from build123d import *

# Parameters (mm, degrees)
BOSS_EXTRUDE1_DEPTH     = 40
SKETCH2_R               = 1.5
CUT_EXTRUDE1_DEPTH      = 1
CUT_EXTRUDE1_DEPTH_BACK = 12
CHAMFER1_SIZE           = 0.2
SKETCH4_R               = 1.5
BOSS_EXTRUDE2_DEPTH     = 6.5
CHAMFER2_SIZE           = 0.6


with BuildPart() as part:
    # Sketch1 → Boss-Extrude1 (new body)
    with BuildSketch(Plane.XY):
        Polygon((2.621170222, 0), (1.310585111, 2.27), (-1.310585111, 2.27), (-2.621170222, 0), (-1.310585111, -2.27), (1.310585111, -2.27), align=None)
    extrude(amount=BOSS_EXTRUDE1_DEPTH)

    # Sketch2 → Cut-Extrude1 (cut, two sides)
    with BuildSketch(Plane.XY.offset(40)) as cut_extrude1_sk:
        Circle(SKETCH2_R)
    extrude(amount=CUT_EXTRUDE1_DEPTH, mode=Mode.SUBTRACT)
    extrude(cut_extrude1_sk.sketch, amount=-CUT_EXTRUDE1_DEPTH_BACK, mode=Mode.SUBTRACT)

    # Sketch3 → Cut-Revolve1 (revolve, cut)
    with BuildSketch(Plane(origin=(0, 0, 0), x_dir=(1, 0, 0), z_dir=(0, 1, 0))):
        Polygon((-2.621170222, -40), (-2.271170222, -40), (-2.621170222, -39.8), align=None)
    revolve(axis=Axis((0, 0, 28), (0, 0, 1)), mode=Mode.SUBTRACT)

    # Chamfer1
    chamfer1_edges = [part.edges().sort_by_distance(p)[0] for p in [
        (-1.5, 0, 40),
    ]]
    chamfer(chamfer1_edges, length=CHAMFER1_SIZE)

    # Sketch4 → Boss-Extrude2 (add)
    with BuildSketch(Plane(origin=(0, 0, 0), x_dir=(-1, 0, 0), z_dir=(0, 0, -1))):
        Circle(SKETCH4_R)
    extrude(amount=BOSS_EXTRUDE2_DEPTH)

    # Chamfer2
    chamfer2_edges = [part.edges().sort_by_distance(p)[0] for p in [
        (1.5, 0, -6.5),
    ]]
    chamfer(chamfer2_edges, length=CHAMFER2_SIZE)


solid = part.part
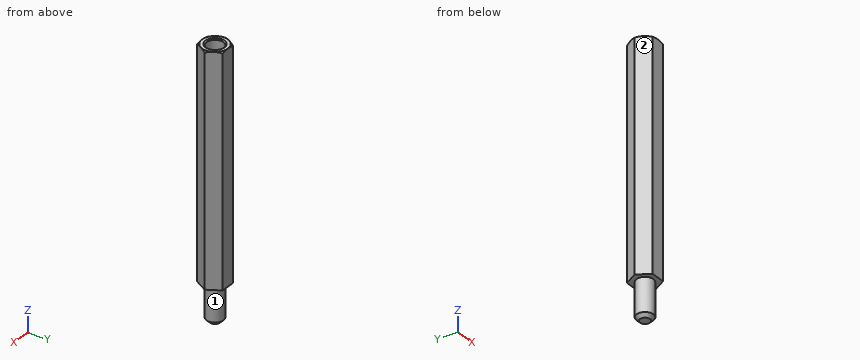
Geometry check sheet. Reference: the model listing, model coordinates, mm. Face numbers are marked on the shaded views. A direction names the side the tool comes from. Coordinates: 2 decimals unless noted, no trailing zeros. Write each loop counter-clockwise with the first axis right and the second up, starting at its lowest first coordinate (ties: lowest second). Pieces come first, ordered by that corner, then holes. Notation, with made-up numbers: (-0.5, -16) -> (27.5, -16) arc R23 cw to (27.5, 17) -> close; hole circle Ø3 at (28.5, 0). An arc over 180 degrees is marked (long way). One line per question, with ' | ' between items.
1. Depth check by flat-ended pin: pin 1 Ø1.5 at (x, y) = (2, -1.5) entering from +Z; pin 2 Ø0.9 at (x, y) = (-0.5, 0) entering from +Z. Enter the tip coordinate at first touch or a pass-through.
Answers:
pin 1: stops at z = 40 | pin 2: stops at z = 28
2. Cross-section at A-A on z = 6. Record the cut outline in (x, y), and give its area (3 significant figures).
Answers:
outline: (-2.62, 0) -> (-1.31, -2.27) -> (1.31, -2.27) -> (2.62, 0) -> (1.31, 2.27) -> (-1.31, 2.27) -> close | area: 17.9 mm²
3. Set-up check for the marked faces 1 and 2: record each of +Z, -Z, +X, -X, +Y, -Y from which the full face is reachable in a straight line by a thin tool's end or side.
Answers:
face 1: -Z | face 2: +Z, -Z, -X, -Y
4. Thickness scan on probe 1 along Y at (x, z) = (0, 30.5); probe 2 along Z at (x, y) = (0.25, 0.45); probe 3 along Z at (x, y) = (0.9, 1.65). Record the ranges inside material, lowest first. Write a range as from..to.
Answers:
probe 1: y = -2.27..-1.5, 1.5..2.27 | probe 2: z = -6.5..28 | probe 3: z = 0..40
